from build123d import *

# Parameters (mm, degrees)
BOSS_EXTRUDE1_DEPTH  = 6
FILLET1_R            = 5
SKETCH2_R            = 2.25
SKETCH2_R_2          = 1.6
CUT_EXTRUDE1_DEPTH   = 123.21292894
FILLET1_OF_MIRROR1_R = 5


with BuildPart() as part:
    # Sketch1 → Boss-Extrude1 (new body)
    with BuildSketch(Plane(origin=(0, 0, 0), x_dir=(1, 0, 0), z_dir=(0, 1, 0))):
        Polygon((-85, 0), (-85, 70), (-100, 70), (-100, -15), (0, -15), (0, 0), (0, 60), (-15, 60), (-15, 0), align=None)
    boss_extrude1 = extrude(amount=BOSS_EXTRUDE1_DEPTH)

    # Fillet1
    fillet1_edges = [part.edges().sort_by_distance(p)[0] for p in [
        (-100, 3, 15),
        (-100, 3, -70),
        (-85, 3, -70),
        (-85, 3, 0),
        (-15, 3, 0),
    ]]
    fillet(fillet1_edges, radius=FILLET1_R)

    # Sketch2 → Cut-Extrude1 (cut, through all)
    with BuildSketch(Plane(origin=(0, 6, 0), x_dir=(1, 0, 0), z_dir=(0, 1, 0))):
        with Locations(Location((-15, -7.5, 0), (0, 0, 270))):
            Circle(SKETCH2_R)
        with Locations(Location((-80, -7.5, 0), (0, 0, 270))):
            Circle(SKETCH2_R_2)
        with Locations(Location((-7.5, 52.5, 0), (0, 0, 270))):
            Circle(SKETCH2_R_2)
    cut_extrude1 = extrude(amount=-CUT_EXTRUDE1_DEPTH, mode=Mode.SUBTRACT)

    # Mirror1: Boss-Extrude1, Cut-Extrude1 across plane
    add(boss_extrude1.mirror(Plane(origin=(0, 0, 0), x_dir=(0, 0, 1), z_dir=(1, 0, 0))))
    add(cut_extrude1.mirror(Plane(origin=(0, 0, 0), x_dir=(0, 0, 1), z_dir=(1, 0, 0))), mode=Mode.SUBTRACT)

    # Fillet1 of Mirror1
    fillet1_of_mirror1_edges = [part.edges().sort_by_distance(p)[0] for p in [
        (100, 3, 15),
        (100, 3, -70),
        (85, 3, -70),
        (85, 3, 0),
        (15, 3, 0),
    ]]
    fillet(fillet1_of_mirror1_edges, radius=FILLET1_OF_MIRROR1_R)


solid = part.part
Here's how the part is built. I have some questions about the finished solid (model axes, mm). A direction names the side the tool comes from. Coordinates: 2 decimals unless noted, no trailing zeros. Order: outer loops, then holes, each group sorted by start corner. A loop starts at its lowest first (then second) coordinate and runs counter-clockwise, first axis right, second up. Notation, with made-up numbers: (19.5, 37) -> (37.5, 37) arc R10 cw to (37.5, 49) -> close; hole circle Ø11 at (-9, -10.5). An arc over 180 degrees is marked (long way). Answer in a Markdown table with one row per item.
(1) On a 3-axis mill with a long thin cutter (end or side, diameter ignored), from which of +Z, -Z, +X, -X, +Y, -Y can I reach the whole of each face in a straight line? I mean faces 1 (the face through (-84, 3, -2)), 2 (the face through (99, 3, 13)). Say none if no direction works.
Answer key:
| item | result |
|---|---|
| face 1 | -Z, +Y, -Y |
| face 2 | +Z, +X, +Y, -Y |
(2) Please list where these lines run through material, in increasing order: probe 1 along X at (y, z) = (0.4, -18); probe 2 along X at (y, z) = (3.5, 7.5); probe 3 along Z at (x, y) = (80, 1.35).
Answer key:
| item | result |
|---|---|
| probe 1 | -100 to -85, -15 to 15, 85 to 100 |
| probe 2 | -100 to -81.6, -78.4 to -17.25, -12.75 to 12.75, 17.25 to 78.4, 81.6 to 100 |
| probe 3 | 0 to 5.9, 9.1 to 15 |
(3) I want a section at D-D on x = 44. List the corners of the cut face in (y, z) for me.
Answer key:
| item | result |
|---|---|
| outline | (0, 0) -> (6, 0) -> (6, 15) -> (0, 15) -> close |
(4) I want a section at B-B on y = 2. List the corners of the cut face in (x, z) for me, then the cut area to 3 significant figures.
Answer key:
| item | result |
|---|---|
| outline | (-100, -65) arc R5 ccw to (-95, -70) -> (-90, -70) arc R5 ccw to (-85, -65) -> (-85, -5) arc R5 cw to (-80, 0) -> (-20, 0) arc R5 cw to (-15, -5) -> (-15, -60) -> (15, -60) -> (15, -5) arc R5 cw to (20, 0) -> (80, 0) arc R5 cw to (85, -5) -> (85, -65) arc R5 ccw to (90, -70) -> (95, -70) arc R5 ccw to (100, -65) -> (100, 10) arc R5 ccw to (95, 15) -> (-95, 15) arc R5 ccw to (-100, 10) -> close; hole circle Ø3.2 at (-80, 7.5); hole circle Ø4.5 at (-15, 7.5); hole circle Ø3.2 at (-7.5, -52.5); hole circle Ø3.2 at (7.5, -52.5); hole circle Ø4.5 at (15, 7.5); hole circle Ø3.2 at (80, 7.5) |
| area | 6,830 mm^2 |
(5) Will these pins go through, and if not, where does the flat tip stop? pin 1 Ø1.8 at (x, y) = (7, 3) entering from -Z; pin 2 Ø4 at (x, z) = (15, 7.5) entering from +Y; pin 3 Ø2 at (x, y) = (-52.5, 1) entering from -Z.
Answer key:
| item | result |
|---|---|
| pin 1 | z = -60 |
| pin 2 | through |
| pin 3 | z = 0 |
(6) I want a section at A-A on z = -32.5. List the corners of the cut face in (x, y) for me.
Answer key:
| item | result |
|---|---|
| outline | (-100, 0) -> (-85, 0) -> (-85, 6) -> (-100, 6) -> close; (-15, 0) -> (15, 0) -> (15, 6) -> (-15, 6) -> close; (85, 0) -> (100, 0) -> (100, 6) -> (85, 6) -> close |
(7) Thinking about a two-plate mould opening in X: for faces 3 (the face through (-100, 3, -28)), 4 (the face through (-86, 3, -68)), 5 (the face through (1, 0, -19)), which applies, +X half, -X half, draft (parallel to the pull), parting line (faces both ways), or undercut?
Answer key:
| item | result |
|---|---|
| face 3 | -X half |
| face 4 | undercut |
| face 5 | draft |
(8) I want a section at C-C on z = -63. List the corners of the cut face in (x, y) for me.
Answer key:
| item | result |
|---|---|
| outline | (-100, 0) -> (-85, 0) -> (-85, 6) -> (-100, 6) -> close; (85, 0) -> (100, 0) -> (100, 6) -> (85, 6) -> close |
